Design review of the part built by this model. Coordinates are the model's own, in mm. A direction names the side the tool comes from. Coordinates: 2 decimals unless noted, no trailing zeros. Loops run counter-clockwise (first coordinate to the right, second up) from the corner with the lowest first, then second, coordinate; pieces in that order, holes last. Notation, with made-up numbers: M 63.25,48.25 L 92.25,48.25 A13 cw 92.25,61.25 Z; hole C 44.25,83.5 d6. An arc over 180 degrees is marked long. One line per item, written item: value.
```python
from build123d import *

# Parameters (mm, degrees)
F1_DEPTH        = 25
F2_R            = 12.5
F3_DEPTH        = 15
F4_W            = 10
F4_H            = 25
F5_DEPTH        = 1.5
F5_COPIES_COUNT = 4


# Not quite as in the source:
# - a pattern or mirror of a feature is missing from the dataset's text; its kind, count and spacing are read off the source's solid


with BuildPart() as f1:
    # F0 (on Top) → F1 (new body)
    with BuildSketch(Plane.XY):
        with BuildLine():
            ThreePointArc((15, -39.0512483795), (15.4733973541, -37.4337567815), (16.7441860465, -36.3267426786))
            ThreePointArc((16.7441860465, -36.3267426786), (0, 40), (-16.7441860465, -36.3267426786))
            ThreePointArc((-16.7441860465, -36.3267426786), (-15.4733973541, -37.4337567815), (-15, -39.0512483795))
            Line((-15, -39.0512483795), (-15, -57))
            ThreePointArc((-15, -57), (-14.1213203436, -59.1213203436), (-12, -60))
            Line((-12, -60), (12, -60))
            ThreePointArc((12, -60), (14.1213203436, -59.1213203436), (15, -57))
            Line((15, -57), (15, -39.0512483795))
        make_face()
    extrude(amount=F1_DEPTH)

    # F2 (on face) → F3 (cut)
    with BuildSketch(Plane.XY.offset(25)):
        Circle(F2_R)
    extrude(amount=-F3_DEPTH, mode=Mode.SUBTRACT)

    # F4 (on Right) → F5 (join, symmetric)
    with BuildSketch(Plane.YZ):
        with Locations((-25, 37.5)):
            Rectangle(F4_W, F4_H)
    f5 = extrude(amount=F5_DEPTH, both=True)

    # F5_copies: F5 ×4 about axis
    f5_copies_axis = Axis((0, 0, 0), (0, 0, 1))
    for i in range(1, F5_COPIES_COUNT):
        add(f5.rotate(f5_copies_axis, i * 360 / F5_COPIES_COUNT))


solid = f1.part
```
(1) Insertion check: pin 1 (0.9 mm diameter, centred on y = 0.5, z = 33, fed in from -X); pin 2 (11 mm diameter, centred on y = 25.5, z = 31.5, fed in from +X); pin 3 (5 mm diameter, centred on x = -27.5, z = 36, fed in from -Y); pin 4 (4 mm diameter, centred on x = 24.5, y = 0.5, fed in from -Z). Each pin has a flat end and moves straight along its axis. Give the tip position at first contact, or say it passes through.
Reply:
pin 1: stops at x = -30
pin 2: stops at x = 1.5
pin 3: stops at y = -1.5
pin 4: stops at z = 0
(2) To check wall thickness, follow line 1 along X through (y, z) = (23, 34.5); line 2 along X through (y, z) = (-52, 14); line 3 along Z through (x, y) = (-23, 4). State the ranges of each line that lie inside material, in increasing order. Write a range as [from, to].
Reply:
line 1: x = [-1.5, 1.5]
line 2: x = [-15, 15]
line 3: z = [0, 25]
(3) Mouldability with a two-part tool opening along X and no side actions: class faces 5 (the flat face through (25, 0, 50)), 6 (the flat face through (20, 0, 37)), 7 (the flat face through (1.5, 25, 38)), 8 (the cylindrical face through (-14.14, -59.1, 12.32)) as released by +X, released by -X, zero draft, split by the parting line, or undercut.
Reply:
face 5: zero draft
face 6: undercut
face 7: released by +X
face 8: released by -X
(4) We need section C-C on y = 0. State the section outline as (x, z) points, then the cut area to 4 significant figures.
Reply:
outline: M -40,0 L 40,0 L 40,25 L 30,25 L 30,50 L 20,50 L 20,25 L 12.5,25 L 12.5,10 L -12.5,10 L -12.5,25 L -20,25 L -20,50 L -30,50 L -30,25 L -40,25 Z
area: 2,125 mm2
(5) Tool access review of faces 1 (the flat face through (0, 20, 37)), 2 (the flat face through (-25, 1.5, 38)), 3 (the flat face through (0, -30, 37)), 4 (the cylindrical face through (11.923, 3.755, 17.605)): name each direction out of +Z, -Z, +X, -X, +Y, -Y from which nothing blocks a thin tool from reaching the whole face with its end or side.
Reply:
face 1: +Z, +X, -X
face 2: +Z, +X, -X, +Y
face 3: +Z, +X, -X, -Y
face 4: +Z
(6) We need section B-B on x = 0. State the section outline as (y, z) points, then the cut area to 4 significant figures.
Reply:
outline: M -60,0 L 40,0 L 40,25 L 30,25 L 30,50 L 20,50 L 20,25 L 12.5,25 L 12.5,10 L -12.5,10 L -12.5,25 L -20,25 L -20,50 L -30,50 L -30,25 L -60,25 Z
area: 2,625 mm2
(7) We need section D-D on x = 18.5. State the section outline as (y, z) points.
Reply:
outline: M -35.46,0 L 35.46,0 L 35.46,25 L -35.46,25 Z
(8) We need section A-A on z = 35.5. State the section outline as (x, y) points.
Reply:
outline: M -30,-1.5 L -20,-1.5 L -20,1.5 L -30,1.5 Z; M -1.5,-30 L 1.5,-30 L 1.5,-20 L -1.5,-20 Z; M -1.5,20 L 1.5,20 L 1.5,30 L -1.5,30 Z; M 20,-1.5 L 30,-1.5 L 30,1.5 L 20,1.5 Z
